Here's how the part is built. I have some questions about the finished solid (model axes, mm). Coordinates: 2 decimals unless noted, no trailing zeros. Write each loop counter-clockwise with the first axis right and the second up, starting at its lowest first coordinate (ties: lowest second). Pieces come first, ordered by that corner, then holes. Notation, with made-up numbers: M 30.25,25 L 52.25,25 A6 cw 52.25,36 Z; hole C 62.5,89 d3. An arc over 180 degrees is marked long. Use a Markdown table: item, result.
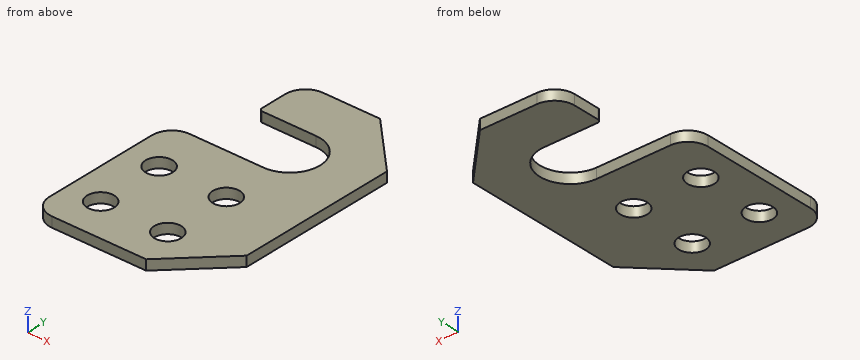
```python
from build123d import *

# Parameters (mm, degrees)
SKETCH1_W           = 30
SKETCH1_H           = 40
SKETCH1_R           = 2
BOSS_EXTRUDE1_DEPTH = 1.5
CHAMFER1_SIZE       = 8
CUT_EXTRUDE1_DEPTH  = 5
FILLET1_R           = 3
FILLET2_R           = 0.5


with BuildPart() as part:
    # Sketch1 → Boss-Extrude1 (new body)
    with BuildSketch(Plane.XY):
        with Locations((15, -20)):
            Rectangle(SKETCH1_W, SKETCH1_H)
        with Locations((20, -34)):
            Circle(SKETCH1_R, mode=Mode.SUBTRACT)
        with Locations((10, -34)):
            Circle(SKETCH1_R, mode=Mode.SUBTRACT)
        with Locations((20, -24)):
            Circle(SKETCH1_R, mode=Mode.SUBTRACT)
        with Locations((10, -24)):
            Circle(SKETCH1_R, mode=Mode.SUBTRACT)
    extrude(amount=BOSS_EXTRUDE1_DEPTH)

    # Chamfer1
    chamfer1_edges = [part.edges().sort_by_distance(p)[0] for p in [
        (30, 0, 0.75),
        (30, -40, 0.75),
    ]]
    chamfer(chamfer1_edges, length=CHAMFER1_SIZE)

    # Sketch2 → Cut-Extrude1 (cut)
    with BuildSketch(Plane.XY.offset(1.5)):
        with BuildLine():
            Line((5, -16.5), (19, -16.5))
            ThreePointArc((19, -16.5), (23.5, -12), (19, -7.5))
            Line((19, -7.5), (10.5, -7.5))
            Line((10.5, -7.5), (10.5, 0))
            Line((10.5, 0), (0, 0))
            Line((0, 0), (0, -16.5))
            Line((0, -16.5), (0, -40))
            Line((0, -40), (5, -40))
            Line((5, -40), (5, -16.5))
        make_face()
    extrude(amount=-CUT_EXTRUDE1_DEPTH, mode=Mode.SUBTRACT)

    # Fillet1
    fillet1_edges = [part.edges().sort_by_distance(p)[0] for p in [
        (10.5, 0, 0.75),
        (5, -40, 0.75),
        (5, -16.5, 0.75),
    ]]
    fillet(fillet1_edges, radius=FILLET1_R)

    # Fillet2
    fillet2_edges = [part.edges().sort_by_distance(p)[0] for p in [
        (10.5, -7.5, 0.75),
    ]]
    fillet(fillet2_edges, radius=FILLET2_R)


solid = part.part
```
1. Suppose I cut it at C-C on z = 0.3. Write out the boundary of the cut face in (x, y), and give its area (3 significant figures).
Answers follow:
| item | result |
|---|---|
| outline | M 5,-37 A3 ccw 8,-40 L 22,-40 L 30,-32 L 30,-8 L 22,0 L 13.5,0 A3 ccw 10.5,-3 L 10.5,-7 A0.5 ccw 11,-7.5 L 19,-7.5 A4.5 cw 19,-16.5 L 8,-16.5 A3 ccw 5,-19.5 Z; hole C 10,-34 d4; hole C 10,-24 d4; hole C 20,-34 d4; hole C 20,-24 d4 |
| area | 681 mm2 |
2. I need wall thicknesses on probe 1 along Y at (x, z) = (14, 1.35); probe 2 along Y at (x, z) = (20, 0.3); probe 3 along Y at (x, z) = (18.25, 1.05). Which ranges of each line are inside material? Lowest first, please.
Answers follow:
| item | result |
|---|---|
| probe 1 | y = -40 to -16.5, -7.5 to 0 |
| probe 2 | y = -40 to -36, -32 to -26, -22 to -16.39, -7.61 to 0 |
| probe 3 | y = -40 to -34.97, -33.03 to -24.97, -23.03 to -16.5, -7.5 to 0 |
3. Suppose I cut it at A-A on y = -34. Write out the boundary of the cut face in (x, z).
Answers follow:
| item | result |
|---|---|
| outline | M 5,0 L 8,0 L 8,1.5 L 5,1.5 Z; M 12,0 L 18,0 L 18,1.5 L 12,1.5 Z; M 22,0 L 28,0 L 28,1.5 L 22,1.5 Z |
4. Will these pins go through, and if not, where does the flat tip stop? pin 1 Ø6.5 at (x, y) = (10, -24) entering from +Z; pin 2 Ø0.8 at (y, z) = (-5, 0.5) entering from -X.
Answers follow:
| item | result |
|---|---|
| pin 1 | stops at z = 1.5 |
| pin 2 | stops at x = 10.5 |
5. Suppose I cut it at B-B on x = 14. Write out the boundary of the cut face in (y, z), and give its area (3 significant figures).
Answers follow:
| item | result |
|---|---|
| outline | M -40,0 L -16.5,0 L -16.5,1.5 L -40,1.5 Z; M -7.5,0 L 0,0 L 0,1.5 L -7.5,1.5 Z |
| area | 46.5 mm2 |
6. Suppose I cut it at D-D on x = 10. Write out the boundary of the cut face in (y, z).
Answers follow:
| item | result |
|---|---|
| outline | M -40,0 L -36,0 L -36,1.5 L -40,1.5 Z; M -32,0 L -26,0 L -26,1.5 L -32,1.5 Z; M -22,0 L -16.5,0 L -16.5,1.5 L -22,1.5 Z |
